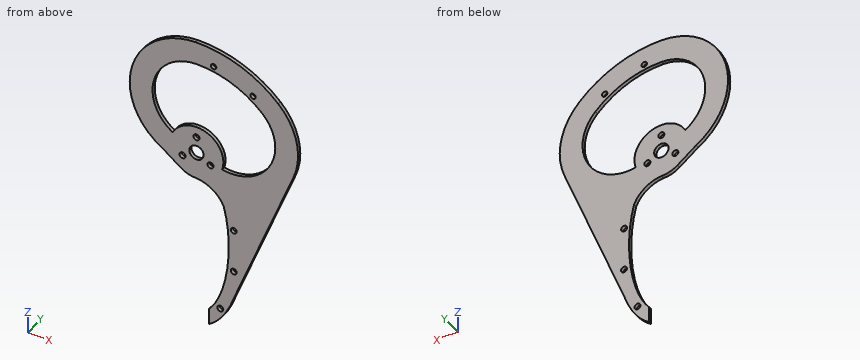
```python
from build123d import *

# Parameters (mm, degrees)
SKETCH_1_R          = 1.5
SKETCH_1_R_2        = 4
SKETCH_1_R_3        = 1.7
EXTRUDE_1_DEPTH     = 2
SKETCH_2_R          = 1.65
CUT_EXTRUDE_1_DEPTH = 114.211457996


with BuildPart() as part:
    # Эскиз1 → Бобышка-Вытянуть1 (new body)
    with BuildSketch(Plane(origin=(0, 0, 0), x_dir=(1, 0, 0), z_dir=(0, 1, 0))):
        with BuildLine():
            Line((53.958573959, -5.561349479), (20.929615764, 77.346018647))
            add(Edge.make_bspline(
                [(20.929615764, 77.346018647), (15.874013102, 92.823492357), (7, 98)],
                knots=[5.291070227, 5.291070227, 5.291070227, 5.999391198, 5.999391198, 5.999391198], degree=2, weights=[1, 0.937937966, 1]))
            Line((7, 98), (7, 89.125236548))
            add(Edge.make_bspline(
                [(15.192612979, 25.829512169), (26.645146253, 67.955139718), (7, 89.125236548)],
                knots=[4.109476107, 4.109476107, 4.109476107, 5.848164932, 5.848164932, 5.848164932], degree=2, weights=[1, 0.645327493, 1]))
            ThreePointArc((15.192612979, 25.829512169), (9.04718601, 18.379331895), (0, 15))
            ThreePointArc((0, 15), (-4.727432256, 14.235567578), (-8.97302418, 12.020184569))
            Line((-8.97302418, 12.020184569), (-19.356829743, 4.268711381))
            ThreePointArc((-19.356829743, 4.268711381), (-35.846538498, -37.448042935), (-0.216613019, -64.70068493))
            ThreePointArc((-0.216613019, -64.70068493), (24.602337984, -59.841043752), (45.662397444, -45.83853195))
            ThreePointArc((45.662397444, -45.83853195), (55.881669425, -26.950465422), (53.958573959, -5.561349479))
        make_face()
        with Locations(Location((9.550649772, -54.164426416, 0), (0, 0, 270))):
            Circle(SKETCH_1_R, mode=Mode.SUBTRACT)
        with Locations(Location((31.546703999, -45.053362436, 0), (0, 0, 90))):
            Circle(SKETCH_1_R, mode=Mode.SUBTRACT)
        with Locations(Location((0, 0, 0), (0, 0, 270))):
            Circle(SKETCH_1_R_2, mode=Mode.SUBTRACT)
        with Locations(Location((0, -9, 0), (0, 0, 270))):
            Circle(SKETCH_1_R_3, mode=Mode.SUBTRACT)
        with Locations(Location((-7.794228634, 4.5, 0), (0, 0, 270))):
            Circle(SKETCH_1_R_3, mode=Mode.SUBTRACT)
        with Locations(Location((7.794228634, 4.5, 0), (0, 0, 270))):
            Circle(SKETCH_1_R_3, mode=Mode.SUBTRACT)
        with BuildLine():
            ThreePointArc((0, -52), (19.899538483, -48.041735691), (36.769552622, -36.769552622))
            ThreePointArc((36.769552622, -36.769552622), (40.965347854, -7.734611808), (14.306107991, 4.50946495))
            ThreePointArc((14.306107991, 4.50946495), (10.606601718, -10.606601718), (-4.50946495, -14.306107991))
            ThreePointArc((-4.50946495, -14.306107991), (-9.64091288, -11.491422838), (-13.304619219, -6.927272727))
            ThreePointArc((-13.304619219, -6.927272727), (-23.497678802, -34.43607172), (0, -52))
        make_face(mode=Mode.SUBTRACT)
    extrude(amount=EXTRUDE_1_DEPTH)

    # Эскиз2 → Вырез-Вытянуть1 (cut, through all)
    with BuildSketch(Plane.XZ):
        with Locations(Location((20.772601242, -38.006933081, 0), (0, 0, 270))):
            Circle(SKETCH_2_R)
        with Locations(Location((13.298587158, -86.537567928, 0), (0, 0, 270))):
            Circle(SKETCH_2_R)
        with Locations(Location((20.772601242, -61.993066919, 0), (0, 0, 270))):
            Circle(SKETCH_2_R)
    extrude(amount=-CUT_EXTRUDE_1_DEPTH, mode=Mode.SUBTRACT)


solid = part.part
```
Check sheet for the modelled part. Datum: model origin and axes. Units: mm. Coordinates: 2 decimals unless noted, no trailing zeros. Write each loop counter-clockwise with the first axis right and the second up, starting at its lowest first coordinate (ties: lowest second). Pieces come first, ordered by that corner, then holes. Notation, with made-up numbers: (6, 3) -> (38, 3) arc R21 ccw to (38, 27) -> close; hole circle Ø3 at (41.25, -14.5). An arc over 180 degrees is marked (long way). Use a Markdown table: item, result.
1. Sectioned sample at B-B (z = 0). Enter the section's corners in (x, y), plus the area to 3 significant figures.
Reported:
| item | result |
|---|---|
| outline | (-25.05, 0) -> (-4, 0) -> (-4, 2) -> (-25.05, 2) -> close; (4, 0) -> (15, 0) -> (15, 2) -> (4, 2) -> close; (34.35, 0) -> (51.74, 0) -> (51.74, 2) -> (34.35, 2) -> close |
| area | 98.9 mm2 |
2. Sectioned sample at A-A (z = 18). Enter the section's corners in (x, y).
Reported:
| item | result |
|---|---|
| outline | (-35.97, 0) -> (-22.58, 0) -> (-22.58, 2) -> (-35.97, 2) -> close; (43.9, 0) -> (56.62, 0) -> (56.62, 2) -> (43.9, 2) -> close |
3. Sectioned sample at C-C (y = 1.2). Give the number of separate pieces and of enclosed holes in the cut face, plus the area to 3 significant figures.
Reported:
| item | result |
|---|---|
| separate pieces | 1 |
| enclosed holes | 10 |
| area | 4,510 mm2 |
4. Sectioned sample at D-D (z = 39). Enter the section's corners in (x, y).
Reported:
| item | result |
|---|---|
| outline | (-35.38, 0) -> (-21.63, 0) -> (-21.63, 2) -> (-35.38, 2) -> close; (34.39, 0) -> (51.09, 0) -> (51.09, 2) -> (34.39, 2) -> close |
5. Scan lines: line 1 along X through (y, z) = (1.5, 0); line 2 along Z through (x, y) = (8.5, 1.65) (3 decimals); line 3 along X through (y, z) = (0.9, -61.5). Record each from-to range of solid material in increasing order.
Reported:
| item | result |
|---|---|
| line 1 | x = -25.05 to -4, 4 to 15, 34.35 to 51.74 |
| line 2 | z = -97.021 to -87.31, -18.004 to -6.047, -2.953 to 12.359, 51.301 to 53.094, 55.235 to 64.14 |
| line 3 | x = 17.21 to 19.2, 22.35 to 27.24 |
6. Go/stop test with a flat-tipped pin: pin 1 Ø1 at (x, y) = (12, 1) entering from -Z. Record where the tip stops, or that it passes through.
Reported:
| item | result |
|---|---|
| pin 1 | stops at z = -94.4 |
